from build123d import *

# Parameters (mm, degrees)
SKETCH1_R               = 50
BOSS_EXTRUDE1_DEPTH     = 10
SKETCH1_3_R             = 4
CUT_EXTRUDE1_DEPTH      = 10
SKETCH1_4_R             = 20
BOSS_EXTRUDE2_DEPTH     = 62.5
SKETCH3_R               = 6.5
CUT_EXTRUDE3_DEPTH      = 63.5
CUT_EXTRUDE3_DEPTH_BACK = 11


with BuildPart() as part:
    # Sketch1 → Boss-Extrude1 (new body)
    with BuildSketch(Plane.XY):
        Circle(SKETCH1_R)
    extrude(amount=-BOSS_EXTRUDE1_DEPTH)

    # Sketch1<3> → Cut-Extrude1 (cut)
    with BuildSketch(Plane.XY):
        with Locations((-35, 0)):
            Circle(SKETCH1_3_R)
        with Locations((17.5, 30.310889132)):
            Circle(SKETCH1_3_R)
        with Locations((17.5, -30.310889132)):
            Circle(SKETCH1_3_R)
    extrude(amount=-CUT_EXTRUDE1_DEPTH, mode=Mode.SUBTRACT)

    # Sketch1<4> → Boss-Extrude2 (add)
    with BuildSketch(Plane.XY):
        with Locations((-1.640921825, 0)):
            Circle(SKETCH1_4_R)
        with BuildLine():
            ThreePointArc((-17.320508076, 2.5), (-17.5, 0), (-17.320508076, -2.5))
            Line((-17.320508076, -2.5), (-14.790199458, -2.5))
            ThreePointArc((-14.790199458, -2.5), (15, 0), (-14.790199458, 2.5))
            Line((-14.790199458, 2.5), (-17.320508076, 2.5))
        make_face(mode=Mode.SUBTRACT)
    extrude(amount=BOSS_EXTRUDE2_DEPTH)

    # Sketch3 → Cut-Extrude3 (cut, two sides)
    with BuildSketch(Plane.XY) as cut_extrude3_sk:
        Circle(SKETCH3_R)
    extrude(amount=CUT_EXTRUDE3_DEPTH, mode=Mode.SUBTRACT)
    extrude(cut_extrude3_sk.sketch, amount=-CUT_EXTRUDE3_DEPTH_BACK, mode=Mode.SUBTRACT)


solid = part.part
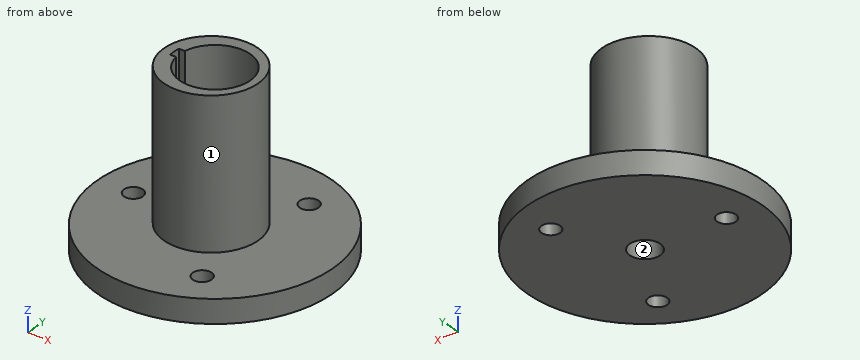
Model file for the job. Use its own axes, mm. Face numbers are marked on the shaded views. A direction names the side the tool comes from. Round coordinates to 2 decimals unless told otherwise and drop trailing zeros. Order: outer loops, then holes, each group sorted by start corner. A loop starts at its lowest first (then second) coordinate and runs counter-clockwise, first axis right, second up.
(1) Pin check, flat tips, straight feed: pin 1 (8 mm diameter, centred on x = 3, y = -6.5, fed in from +Z); pin 2 (7 mm diameter, centred on x = 17.5, y = -30.31, fed in from -Z); pin 3 (2 mm diameter, centred on y = -12, z = 42.5, fed in from -X); pin 4 (1.3 mm diameter, centred on x = -16.5, z = 46.5, fed in from -Y). Stop position of each tip, or through.
(2) Band-saw the part on D-D (y = 28). List the corners of the cut face in (x, z).
(3) Band-saw the part on C-C (x = -35). List the corners of the cut face in (y, z).
(4) Drill centre lines: line 1 (Y direction, x = 17.5, z = -1.75); line 2 (Y direction, x = 0, z = -2); line 3 (Z direction, x = -27.5, y = 7.5). Where is each one in solid material? Low to high.
(5) 3-axis set-ups, long thin cutter, end or side, ignore diameter. For the marked faces 1 and 2: which of +Z, -Z, +X, -X, +Y, -Y reach the whole face in a straight line?
(6) Band-saw the part on A-A (y = 0). List the corners of the cut face in (x, z).
(7) Band-saw the part on B-B (z = 54). List the corners of the cut face in (x, y), then the cut area to 3 significant figures.
Verdict:
1. pin 1: stops at z = 0
1. pin 2: passes through
1. pin 3: stops at x = -18.34
1. pin 4: stops at y = -14.07
2. outline: (-41.42, -10) - (14.24, -10) - (14.24, 0) - (-41.42, 0) - close; (20.76, -10) - (41.42, -10) - (41.42, 0) - (20.76, 0) - close
3. outline: (-35.71, -10) - (-4, -10) - (-4, 0) - (-35.71, 0) - close; (4, -10) - (35.71, -10) - (35.71, 0) - (4, 0) - close
4. line 1: y = -46.84 to -34.31, -26.31 to 26.31, 34.31 to 46.84
4. line 2: y = -50 to -6.5, 6.5 to 50
4. line 3: z = -10 to 0
5. face 1: +Z
5. face 2: +Z, -Z
6. outline: (-50, -10) - (-39, -10) - (-39, 0) - (-50, 0) - close; (-31, -10) - (-6.5, -10) - (-6.5, 0) - (-17.5, 0) - (-17.5, 62.5) - (-21.64, 62.5) - (-21.64, 0) - (-31, 0) - close; (6.5, -10) - (50, -10) - (50, 0) - (18.36, 0) - (18.36, 62.5) - (15, 62.5) - (15, 0) - (6.5, 0) - close
7. outline: circle Ø40 at (-1.64, 0); hole (-17.32, -2.5) - (-14.79, -2.5) arc R15 ccw (long way) to (-14.79, 2.5) - (-17.32, 2.5) arc R17.5 ccw to start
7. area: 537 mm2
